Read the model definition and answer for the solid it produces. Units are mm, in the model's axes. Face numbers are marked on the shaded views. A direction names the side the tool comes from. Coordinates: 2 decimals unless noted, no trailing zeros. Loops run counter-clockwise (first coordinate to the right, second up) from the corner with the lowest first, then second, coordinate; pieces in that order, holes last. Notation, with made-up numbers: (8, 20) - (13, 20) arc R12 cw to (13, 40) - close; hole circle Ø8 at (48.25, 65.5). An arc over 180 degrees is marked (long way). Use one line per item in the form item = value. Start each with the question number.
1) A cutting plane is placed at A-A (x = -46.5). Give the vertices of the cut face in (y, z), and give its area (3 significant figures).
2) Consider line 1 (Z direction, x = -15, y = -26.5); line 2 (Y direction, x = 79, z = -18); line 3 (X direction, y = -9.5, z = -4.5). Determine where each line is inside the solid, lowest interval first.
3) Which of the six approach directions +Z, -Z, +X, -X, +Y, -Y give full straight-line access (tool end or side, diameter ignored) to the marked faces 1 and 2?
4) The mould has two halves that part along X. Classify the marked faces 3, 4 and 5: released by +X, released by -X, zero draft, split by the parting line, or undercut.
5) Each of these flat-tipped pins is pushed along its axis until it touches: P1, Ø10, axis at x = 41.5, z = -16.5, coming from the +Y side; P2, Ø3, axis at y = 4, z = -17, coming from the -X side; P3, Ø12, axis at x = 69.5, y = -14, coming from the +Z side; P4, Ø4, axis at x = 86.5, z = -22.5, coming from the -Y side. Where does it stop, or does it pass through?
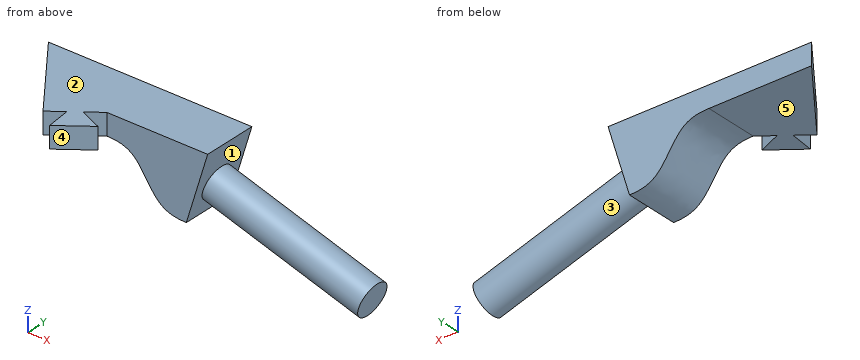
from build123d import *

# Parameters (mm, degrees)
BOSS_EXTRUDE1_DEPTH      = 12.7
BOSS_EXTRUDE1_DEPTH_BACK = 19.878167
SKETCH1_W                = 76.2
SKETCH1_H                = 25.4
CUT_EXTRUDE1_DEPTH       = 50.919049703
SKETCH4_R                = 7.9375
BOSS_EXTRUDE2_DEPTH      = 76.2
BOSS_EXTRUDE3_DEPTH      = 10


with BuildPart() as part:
    # Sketch1 → Boss-Extrude1 (new, two sides: drawn at the far end of the back side and taken through both)
    with BuildSketch(Plane.XY.offset(-BOSS_EXTRUDE1_DEPTH_BACK)):
        Rectangle(SKETCH1_W, SKETCH1_H)
    extrude(amount=BOSS_EXTRUDE1_DEPTH + BOSS_EXTRUDE1_DEPTH_BACK)

    # Sketch2 → Cut-Extrude1 (cut, through all)
    with BuildSketch(Plane.XZ.offset(12.7)):
        Polygon((33.097822487, -3.5890835), (28.095644974, -19.878167), (30.299971912, -19.878167), (38.1, -19.878167), (38.1, -5.125190787), align=None)
        Polygon((38.1, 12.7), (33.097822487, -3.5890835), (38.1, -5.125190787), align=None)
        with BuildLine():
            Line((28.095644974, -19.878167), (-38.1, -19.878167))
            Line((-38.1, -19.878167), (-38.1, 2.7))
            Line((-38.1, 2.7), (-9.105646135, 2.7))
            add(Edge.make_bspline(
                [(28.095644974, -19.878167), (23.262476233, -19.878167), (13.759725723, -18.38827049), (5.19295176, 1.21010349), (-4.185142014, 2.7), (-9.105646135, 2.7)],
                knots=[0, 0, 0, 0, 0.311689084, 0.688310916, 1, 1, 1, 1], degree=3))
        make_face()
    extrude(amount=-CUT_EXTRUDE1_DEPTH, mode=Mode.SUBTRACT)

    # Sketch4 → Boss-Extrude2 (add)
    with BuildSketch(Plane(origin=(31.252760971, 0, -9.59733911), x_dir=(-0.2935578385035089, 0, -0.95594131381228), z_dir=(0.95594131381228, 0, -0.2935578385035089))):
        with Locations((-2.530674188, 0)):
            Circle(SKETCH4_R)
    extrude(amount=BOSS_EXTRUDE2_DEPTH)

    # Sketch5 → Boss-Extrude3 (add)
    with BuildSketch(Plane(origin=(0, 0, 2.7), x_dir=(-1, 0, 0), z_dir=(0, 0, -1))):
        Polygon((38.1, 12.7), (38.1, -12.7), (57.150604496, 12.7), align=None)
        Polygon((27.661608652, -26.617413502), (38.1, -12.7), (9.105646135, -12.7), (16.030761987, -17.894001701), (5.322904607, -22.467747821), (19.34354444, -32.983561373), (20.7364928, -21.423411802), align=None)
    extrude(amount=-BOSS_EXTRUDE3_DEPTH)


solid = part.part
Found:
q1.outline = (-1.5, 2.7) - (12.7, 2.7) - (12.7, 12.7) - (-1.5, 12.7) - close
q1.area = 142 mm^2
q2.line_1 = 2.7 to 12.7
q2.line_2 = -7.15 to 7.15
q2.line_3 = 6.62 to 32.82
q3.face_1 = none
q3.face_2 = +Z, +X, -X, +Y, -Y
q4.face_3 = undercut
q4.face_4 = released by +X
q4.face_5 = zero draft
q5.P1 = 7.86
q5.P2 = 14.78
q5.P3 = through
q5.P4 = -7.94
